Geometry: final body of the model. Coordinates: model frame, mm. A direction names the side the tool comes from. Give positions to 0.01 mm unless a question says otherwise; leave off trailing zeros. Write each loop counter-clockwise with the first axis right and the second up, starting at its lowest first coordinate (ties: lowest second). Pieces come first, ordered by that corner, then holes. Notation, with made-up numbers: (65.5, -1.75) - (96.5, -1.75) arc R31 ccw to (96.5, 36.25) - close; hole circle Ø8 at (17.25, -20). An arc over 180 degrees is marked (long way). Return JSON: item names as keys, results as strings.
from build123d import *

# Parameters (mm, degrees)
EXTRUDE_1_DEPTH     = 102
SKETCH_2_W          = 9
SKETCH_2_H          = 50
EXTRUDE_2_DEPTH     = 6
SKETCH_3_R          = 0.5
SKETCH_3_R_2        = 2.5
CUT_EXTRUDE_1_DEPTH = 10


with BuildPart() as part:
    # 草图1 → 凸台-拉伸1 (new, symmetric)
    with BuildSketch(Plane(origin=(0, 0, 0), x_dir=(0, 0, -1), z_dir=(1, 0, 0))):
        Polygon((-3, 0), (-3, 70), (3, 70), (3, 0), (3, -3.5), (-3, -3.5), align=None)
    extrude(amount=EXTRUDE_1_DEPTH, both=True)

    # 草图2 → 凸台-拉伸2 (add)
    with BuildSketch(Plane(origin=(0, 0, -3), x_dir=(-1, 0, 0), z_dir=(0, 0, -1))):
        with Locations((106.5, 45)):
            Rectangle(SKETCH_2_W, SKETCH_2_H)
    extrude_2 = extrude(amount=-EXTRUDE_2_DEPTH)

    # 草图3 → 切除-拉伸1 (cut)
    with BuildSketch(Plane.ZY.offset(102)):
        with Locations((0, 17)):
            Circle(SKETCH_3_R)
        Circle(SKETCH_3_R_2)
        with Locations((0, 13)):
            Circle(SKETCH_3_R)
        with Locations((0, 9)):
            Circle(SKETCH_3_R)
    cut_extrude_1 = extrude(amount=-CUT_EXTRUDE_1_DEPTH, mode=Mode.SUBTRACT)

    # 镜向1: 凸台-拉伸2, 切除-拉伸1 across plane
    add(extrude_2.mirror(Plane(origin=(0, 0, 0), x_dir=(0, 0, 1), z_dir=(1, 0, 0))))
    add(cut_extrude_1.mirror(Plane(origin=(0, 0, 0), x_dir=(0, 0, 1), z_dir=(1, 0, 0))), mode=Mode.SUBTRACT)


solid = part.part
Q1. Mould query, pull axis Y, two halves, no side actions, for faces 5 (the flat face through (111, 45, 0)), 6 (the flat face through (1, -3.5, 0)), 7 (the cylindrical face through (97.07, -2.44, -0.54)). Classes: pulls with the +Y half, pulls with the -Y half, needs draft (parallel to the pull), parting line crosses it, or undercut.
Answer key:
{"face 5": "needs draft", "face 6": "pulls with the -Y half", "face 7": "undercut"}
Q2. Set-up query: faces 1 (the cylindrical face through (-97.07, -2.44, -0.54)), 2 (the flat face through (92, 0, 0)), 3 (the flat face through (-106, 20, 0)), 4 (the flat face through (106, 20, 0)). Return all of +Z, -Z, +X, -X, +Y, -Y with unobstructed straight access to the full face (end or side cutting, diameter ignored); none if empty.
Answer key:
{"face 1": "-X", "face 2": "+X", "face 3": "+Z, -Z, -X, -Y", "face 4": "+Z, -Z, +X, -Y"}
Q3. Material intervals for probe 1 along Y at (x, z) = (-100, 0); probe 2 along X at (y, z) = (19, 2.75); probe 3 along Y at (x, z) = (-92.5, 1.4), sorted ascending. Write a range as [from, to].
Answer key:
{"probe 1": "y = [-3.5, -2.5], [2.5, 8.5], [9.5, 12.5], [13.5, 16.5], [17.5, 70]", "probe 2": "x = [-102, 102]", "probe 3": "y = [-3.5, -2.07], [2.07, 70]"}
Q4. Pin query (flat end, axial travel): P1, Ø0.5, axis at y = 9, z = 0, coming from the -X side; P2, Ø1.1, axis at y = 13, z = 0, coming from the +X side; P3, Ø3, axis at x = -105.5, z = -1.5, coming from the -Y side. Return the tip coordinate at first contact, or that it passes through.
Answer key:
{"P1": "stops at x = -92", "P2": "stops at x = 102", "P3": "stops at y = 20"}
Q5. Section query A-A, the plane y = 0. Return the cut outline in (x, z), plus the area to 3 significant figures.
Answer key:
{"outline": "(-102, -3) - (102, -3) - (102, -2.5) - (92, -2.5) - (92, 2.5) - (102, 2.5) - (102, 3) - (-102, 3) - (-102, 2.5) - (-92, 2.5) - (-92, -2.5) - (-102, -2.5) - close", "area": "1,120 mm^2"}
